```python
from build123d import *

# Parameters (mm, degrees)
SKETCH_1_W           = 150
SKETCH_1_H           = 90
EXTRUDE_1_DEPTH      = 5
SKETCH_3_R           = 27
CUT_EXTRUDE_1_DEPTH  = 5
SKETCH_4_R           = 2.15
CUT_EXTRUDE_2_DEPTH  = 88.60707734
SKETCH_5_R           = 7.7
CUT_EXTRUDE_3_DEPTH  = 88.60707734
CHAMFER_1_SIZE       = 40
CHAMFER_3_SIZE       = 50
CHAMFER_3_SIZE2      = 41.954981559
CUT_EXTRUDE_4_DEPTH  = 88.60707734
SKETCH_7_W           = 19
SKETCH_7_H           = 30
EXTRUDE_2_DEPTH      = 5
CHAMFER_2_SIZE       = 10
SKETCH_8_R           = 1.65
CUT_EXTRUDE_5_DEPTH  = 105.335995706
SKETCH_10_R          = 1.7
CUT_EXTRUDE_6_DEPTH  = 105.335995706
SKETCH_11_R          = 1.7
CUT_EXTRUDE_7_DEPTH  = 105.335995706
CUT_EXTRUDE_9_DEPTH  = 105.335995706
EXTRUDE_1_2_DEPTH    = 5
CUT_EXTRUDE_10_DEPTH = 105.335995706
FILLET_1_R           = 2
FILLET_2_R           = 4
SKETCH_16_W          = 68
SKETCH_16_H          = 5
EXTRUDE_3_DEPTH      = 3
EXTRUDE_4_DEPTH      = 5
FILLET_3_R           = 1
SKETCH_18_R          = 1.7
CUT_EXTRUDE_11_DEPTH = 106.664563735


with BuildPart() as part:
    # 草图1 → Extrude 1 (new body)
    with BuildSketch(Plane.XY):
        Rectangle(SKETCH_1_W, SKETCH_1_H)
    extrude(amount=EXTRUDE_1_DEPTH)

    # 草图3 → 切除-拉伸1 (cut)
    with BuildSketch(Plane.XY.offset(5)):
        Circle(SKETCH_3_R)
    extrude(amount=-CUT_EXTRUDE_1_DEPTH, mode=Mode.SUBTRACT)

    # 草图4 → 切除-拉伸2 (cut, through all)
    with BuildSketch(Plane.XY.offset(5)):
        with Locations((16.5, 28.578838325)):
            Circle(SKETCH_4_R)
        with Locations((33, 0)):
            Circle(SKETCH_4_R)
        with Locations((16.5, -28.578838325)):
            Circle(SKETCH_4_R)
        with Locations((-16.5, -28.578838325)):
            Circle(SKETCH_4_R)
        with Locations((-33, 0)):
            Circle(SKETCH_4_R)
        with Locations((-16.5, 28.578838325)):
            Circle(SKETCH_4_R)
    extrude(amount=-CUT_EXTRUDE_2_DEPTH, mode=Mode.SUBTRACT)

    # 草图5 → 切除-拉伸3 (cut, through all)
    with BuildSketch(Plane.XY.offset(5)):
        with Locations((57.590256339, 33.24975)):
            Circle(SKETCH_5_R)
    extrude(amount=-CUT_EXTRUDE_3_DEPTH, mode=Mode.SUBTRACT)

    # 倒角1
    chamfer_1_edges = [part.edges().sort_by_distance(p)[0] for p in [
        (75, -45, 2.5),
    ]]
    chamfer(chamfer_1_edges, length=CHAMFER_1_SIZE)

    # 倒角3
    chamfer_3_edges = [part.edges().sort_by_distance(p)[0] for p in [
        (-75, -45, 2.5),
    ]]
    chamfer_3_side = [part.faces().sort_by_distance(p)[0] for p in [
        (-75, 0, 2.5),
    ]]
    chamfer(chamfer_3_edges, length=CHAMFER_3_SIZE, length2=CHAMFER_3_SIZE2, reference=chamfer_3_side[0])

    # 草图6 → 切除-拉伸4 (cut, through all)
    with BuildSketch(Plane(origin=(0, 0, 0), x_dir=(-1, 0, 0), z_dir=(0, 0, -1))):
        Polygon((-39.037333413, -40.962666587), (-35, -40.962666587), (-35, -45), align=None)
        Polygon((36.432743419, -40.962666587), (33.045018441, -40.962666587), (33.045018441, -45), align=None)
    extrude(amount=-CUT_EXTRUDE_4_DEPTH, mode=Mode.SUBTRACT)

    # 草图7 → 凸台-拉伸2 (add, through all)
    with BuildSketch(Plane.XY.offset(5)):
        with Locations((84.5, 30)):
            Rectangle(SKETCH_7_W, SKETCH_7_H)
    extrude(amount=-EXTRUDE_2_DEPTH)

    # 倒角2
    chamfer_2_edges = [part.edges().sort_by_distance(p)[0] for p in [
        (75, 15, 2.5),
    ]]
    chamfer(chamfer_2_edges, length=CHAMFER_2_SIZE)

    # 草图8 → 切除-拉伸5 (cut, through all)
    with BuildSketch(Plane.XY.offset(5)):
        with Locations((90, 19)):
            Circle(SKETCH_8_R)
        with Locations((90, 41)):
            Circle(SKETCH_8_R)
        with Locations((45, 41)):
            Circle(SKETCH_8_R)
        with Locations((45, 19)):
            Circle(SKETCH_8_R)
    extrude(amount=-CUT_EXTRUDE_5_DEPTH, mode=Mode.SUBTRACT)

    # 草图10 → 切除-拉伸6 (cut, through all)
    with BuildSketch(Plane.XY.offset(5)):
        with Locations((-37.348548138, -35.204081542)):
            Circle(SKETCH_10_R)
        with Locations((-43.776424235, -27.543637111)):
            Circle(SKETCH_10_R)
        with Locations((-72, 36.5)):
            Circle(SKETCH_10_R)
        with Locations((-72, 26.5)):
            Circle(SKETCH_10_R)
        with Locations((-69.487928622, 3.098140613)):
            Circle(SKETCH_10_R)
        with Locations((-63.060052525, -4.562303818)):
            Circle(SKETCH_10_R)
    extrude(amount=-CUT_EXTRUDE_6_DEPTH, mode=Mode.SUBTRACT)

    # 草图11 → 切除-拉伸7 (cut, through all)
    with BuildSketch(Plane.XY.offset(5)):
        with Locations((-47, 42)):
            Circle(SKETCH_11_R)
        with Locations((-57, 42)):
            Circle(SKETCH_11_R)
        with Locations((18, 42)):
            Circle(SKETCH_11_R)
        with Locations((28, 42)):
            Circle(SKETCH_11_R)
    extrude(amount=-CUT_EXTRUDE_7_DEPTH, mode=Mode.SUBTRACT)

    # 草图13 → 切除-拉伸9 (cut, through all)
    with BuildSketch(Plane.XY.offset(5)):
        with BuildLine():
            Line((-65, 35), (-65, 8.639702343))
            Line((-65, 8.639702343), (-39.185066827, -22.125337008))
            ThreePointArc((-39.185066827, -22.125337008), (-44.202419924, 8.434813149), (-28.284271247, 35))
            Line((-28.284271247, 35), (-65, 35))
        make_face()
        with BuildLine():
            Line((34.954981559, -28.339888218), (34.954981559, -45))
            Line((34.954981559, -45), (35, -45))
            Line((35, -45), (85, -3.384776311))
            Line((85, -3.384776311), (85, 15))
            Line((85, 15), (42.426406871, 15))
            ThreePointArc((42.426406871, 15), (44.345871246, -7.644848165), (34.954981559, -28.339888218))
        make_face()
    extrude(amount=-CUT_EXTRUDE_9_DEPTH, mode=Mode.SUBTRACT)

    # 草图14 → Extrude 1 2 (add, through all)
    with BuildSketch(Plane.XY.offset(5)):
        Polygon((34.954981559, -28.339888218), (84, 15), (80.689106292, 18.746729621), (31.644087851, -24.593158597), align=None)
    extrude(amount=-EXTRUDE_1_2_DEPTH)

    # 草图15 → 切除-拉伸10 (cut, through all)
    with BuildSketch(Plane.XY.offset(5)):
        with BuildLine():
            Line((64.368429023, 21), (85, 21))
            Line((85, 21), (85, 40))
            Line((85, 40), (69.855415324, 40))
            ThreePointArc((69.855415324, 40), (71.040613965, 29.365437998), (64.368429023, 21))
        make_face()
        with BuildLine():
            Line((25.403039136, 37.144119355), (43.874708376, 36.057550576))
            ThreePointArc((43.874708376, 36.057550576), (44.31250452, 28.811134605), (48.320539762, 22.758212716))
            ThreePointArc((48.320539762, 22.758212716), (43.557063519, 23.802924259), (40.158036561, 20.305962168))
            ThreePointArc((40.158036561, 20.305962168), (33.844416763, 29.657300181), (25.403039136, 37.144119355))
        make_face()
    extrude(amount=-CUT_EXTRUDE_10_DEPTH, mode=Mode.SUBTRACT)

    # 圆角1
    fillet_1_edges = [part.edges().sort_by_distance(p)[0] for p in [
        (64.368429023, 21, 2.5),
        (69.855415324, 40, 2.5),
        (85, 40, 2.5),
        (85, 21, 2.5),
        (40.158036561, 20.305962168, 2.5),
        (25.403039136, 37.144119355, 2.5),
        (43.874708376, 36.057550576, 2.5),
        (48.320539762, 22.758212716, 2.5),
    ]]
    fillet(fillet_1_edges, radius=FILLET_1_R)

    # 圆角2
    fillet_2_edges = [part.edges().sort_by_distance(p)[0] for p in [
        (-65, 35, 2.5),
        (-28.284271247, 35, 2.5),
        (-39.185066827, -22.125337008, 2.5),
        (-65, 8.639702343, 2.5),
        (42.426406871, 15, 2.5),
        (42.392765926, -15.094813585, 2.5),
        (76.449168652, 15, 2.5),
    ]]
    fillet(fillet_2_edges, radius=FILLET_2_R)

    # 草图16 → 凸台-拉伸3 (add)
    with BuildSketch(Plane.XZ.offset(45)):
        with Locations((0.954981559, 2.5)):
            Rectangle(SKETCH_16_W, SKETCH_16_H)
    extrude(amount=EXTRUDE_3_DEPTH)

    # 草图17 → 凸台-拉伸4 (add, through all)
    with BuildSketch(Plane.XY.offset(5)):
        Polygon((-36.432743419, -40.962666587), (-33.045018441, -45), (-33.045018441, -40.962666587), align=None)
    extrude(amount=-EXTRUDE_4_DEPTH)

    # 圆角3
    fillet_3_edges = [part.edges().sort_by_distance(p)[0] for p in [
        (34.954981559, -28.339888218, 2.5),
        (84, 15, 2.5),
        (34.954981559, -48, 2.5),
        (-33.045018441, -48, 2.5),
        (-33.045018441, -45, 2.5),
        (-75, 5, 2.5),
        (-75, 45, 2.5),
        (94, 45, 2.5),
        (94, 15, 2.5),
    ]]
    fillet(fillet_3_edges, radius=FILLET_3_R)

    # 草图18 → 切除-拉伸11 (cut, through all)
    with BuildSketch(Plane.XY.offset(5)):
        with Locations((24.954981559, -45)):
            Circle(SKETCH_18_R)
        with Locations((14.954981559, -45)):
            Circle(SKETCH_18_R)
        with Locations((-13.045018441, -45)):
            Circle(SKETCH_18_R)
        with Locations((-23.045018441, -45)):
            Circle(SKETCH_18_R)
    extrude(amount=-CUT_EXTRUDE_11_DEPTH, mode=Mode.SUBTRACT)


solid = part.part
```
For this review, take the finished solid that the model builds, in its own axes (mm). A direction names the side the tool comes from. Coordinates: 2 decimals unless noted, no trailing zeros. Loops run counter-clockwise (first coordinate to the right, second up) from the corner with the lowest first, then second, coordinate; pieces in that order, holes last. Notation, with made-up numbers: (18, 61.5) - (34, 61.5) arc R32 cw to (34, 92.5) - close; hole circle Ø4 at (-9.5, -35.5). An arc over 180 degrees is marked (long way). Use one line per item in the form item = value. Start each with the question number.
1) Take a section at B-B (y = 19). State the section outline as (x, z) points, plus the area to 3 significant figures.
2) To check wall thickness, follow probe 1 along Y at (x, z) = (-72, 1.7); probe 2 along Y at (x, z) = (0, 1.2); probe 3 along X at (y, z) = (-30, 0.95). State the ranges of each line that lie inside material, in increasing order. Write a range as from..to.
3) Take a section at C-C (z = 4.2). State how many separate pieces and enclosed holes the cut face has, plus the area to 3 significant figures.
4) For faces 4 (the face through (-75, 24, 2)), 5 (the face through (69.646, 12.353, 2.465)), list the 3-axis set-ups (+Z, -Z, +X, -X, +Y, -Y) from which the entire face can be reached by the end or side of a thin tool; tool diameter is ignored.
5) Draft analysis for pull direction Y (two halves, no side actions). For faces 1 (the face through (8, 30, 5)), 2 (the face through (-49, 35, 3)), 3 (the face through (0, -48, 3)), state which applies: released by +Y, released by -Y, zero draft, split by the parting line, or undercut.
6) Take a section at A-A (x = 0). State the section outline as (y, z) points.
7) For pin 1 (3 mm diameter, centred on x = -47, y = 42, fed in from -Z); pin 2 (1 mm diameter, centred on y = -8.5, z = 2, fed in from +X), all flat-tipped, find the tip position at first contact; note any pin that passes through.
From the geometry:
q1.outline = (-75, 0) - (-65, 0) - (-65, 5) - (-75, 5) - close; (-40.79, 0) - (-19.18, 0) - (-19.18, 5) - (-40.79, 5) - close; (19.18, 0) - (43.35, 0) - (43.35, 5) - (19.18, 5) - close; (46.65, 0) - (88.35, 0) - (88.35, 5) - (46.65, 5) - close; (91.65, 0) - (94, 0) - (94, 5) - (91.65, 5) - close
q1.area = 499 mm2
q2.probe_1 = 1.42..24.8, 28.2..34.8, 38.2..45
q2.probe_2 = -48..-27, 27..45
q2.probe_3 = -45.63..-18.11, -14.89..14.89, 18.11..34.95
q3.separate_pieces = 1
q3.enclosed_holes = 30
q3.area = 7,440 mm2
q4.face_4 = +Z, -Z, -X, +Y, -Y
q4.face_5 = +Z, -Z
q5.face_1 = zero draft
q5.face_2 = undercut
q5.face_3 = released by -Y
q6.outline = (-48, 0) - (-27, 0) - (-27, 5) - (-48, 5) - close; (27, 0) - (45, 0) - (45, 5) - (27, 5) - close
q7.pin_1 = through
q7.pin_2 = 57.97
